The drawing under review shows one solid part. Ordinate dimensions are in mm from its lowest x, y, z. A direction names the side the tool comes from. Round coordinates to 2 decimals unless told otherwise and drop trailing zeros. Write each loop counter-clockwise with the first axis right and the second up, starting at its lowest first coordinate (ties: lowest second). Pieces come first, ordered by that corner, then holes. Notation, with made-up numbers: M -24.5,-1 L -7.5,-1 A37 cw -7.5,36 Z; hole C 48,13.5 d6. An arc over 180 degrees is marked long. Write item = value, one per line. Start each with the question number.
Item 1: Take a section at A-A, the plane z = 10. Give the boundary of the cut face in (x, y), plus the area to 3 significant figures.
Item 2: Take a section at B-B, the plane x = 9. Give the boundary of the cut face in (y, z), plus the area to 3 significant figures.
Item 3: Take a section at C-C, the plane y = 7.5. Give the boundary of the cut face in (x, z).
Item 4: To check wall thickness, follow line 1 along X through (y, z) = (3, 10); line 2 along X through (y, z) = (5.5, 10); line 3 along Y through (x, z) = (17, 13). State the ranges of each line that lie inside material, in increasing order.
Item 5: For pin 1 Ø4.5 at (x, z) = (10, 10) entering from -Y; pin 2 Ø4 at (y, z) = (3, 7) entering from -X; pin 3 Ø6 at (x, y) = (17, 9) entering from -Z; pin 4 Ø3 at (y, z) = (9.5, 3.5) entering from +X, all flat-tipped, find the tip position at first contact; note any pin that passes through.
Item 6: Tool access review of the marked faces 4 and 5: name each direction out of +Z, -Z, +X, -X, +Y, -Y from which nothing blocks a thin tool from reaching the whole face with its end or side.
Item 7: Take a section at D-D, the plane z = 5.5. Give the boundary of the cut face in (x, y).
Item 8: The part is to be moulded in two halves that separate along Z. For the marked faces 1, 2 and 3, say which applies: +Z half, -Z half, draft (parallel to the pull), parting line (faces both ways), or undercut.
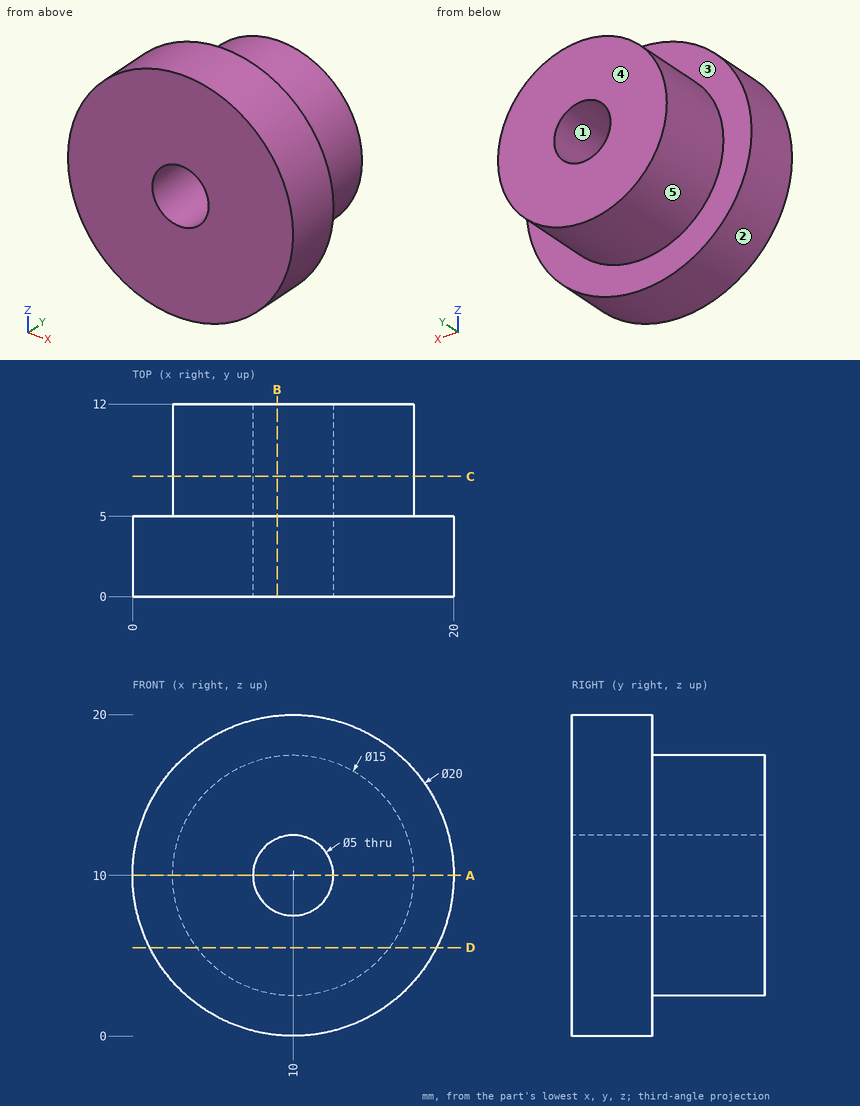
Response values:
q1.outline = M 0,0 L 7.5,0 L 7.5,12 L 2.5,12 L 2.5,5 L 0,5 Z; M 12.5,0 L 20,0 L 20,5 L 17.5,5 L 17.5,12 L 12.5,12 Z
q1.area = 145 mm2
q2.outline = M 0,0.05 L 5,0.05 L 5,2.57 L 12,2.57 L 12,7.71 L 0,7.71 Z; M 0,12.29 L 12,12.29 L 12,17.43 L 5,17.43 L 5,19.95 L 0,19.95 Z
q2.area = 149 mm2
q3.outline = C 10,10 d15; hole C 10,10 d5
q4.line_1 = 0 to 7.5, 12.5 to 20
q4.line_2 = 2.5 to 7.5, 12.5 to 17.5
q4.line_3 = 0 to 5
q5.pin_1 = through
q5.pin_2 = 0.05
q5.pin_3 = 3.66
q5.pin_4 = 15.59
q6.face_4 = +Z, -Z, +X, -X, +Y
q6.face_5 = +Y
q7.outline = M 1.07,0 L 18.93,0 L 18.93,5 L 16,5 L 16,12 L 4,12 L 4,5 L 1.07,5 Z
q8.face_1 = undercut
q8.face_2 = parting line
q8.face_3 = draft
